Autodesk Inventor part; units mm, degrees
ref_plane "YZ Plane" through (0, 0, 0) normal (1, 0, 0) x (0, 1, 0)
ref_plane "XZ Plane" through (0, 0, 0) normal (0, 1, 0) x (-1, 0, 0)
ref_plane "XY Plane" through (0, 0, 0) normal (0, 0, 1) x (1, 0, 0)
sketch "Skizze1" plane through (0, 0, 0) normal (0, 1, 0) x (-1, 0, 0)
  line L0 (31, 31) -> (-31, 31)
  line L1 (-31, 31) -> (-31, -31)
  line L2 (-31, -31) -> (31, -31)
  line L3 (31, -31) -> (31, 31)
  line L4 (31, 31) -> (-31, -31) construction
  line L5 (-31, 31) -> (31, -31) construction
  point P0 (0, 0)
  dimension "d0" = 62
  dimension "d1" = 62
extrude "Extrusion1" add sketch "Skizze1" along normal blind 2
fillet "Rundung1" radius 6 4 edges at (-31, 1, 31) (31, 1, 31) (31, 1, -31) (-31, 1, -31)
sketch "Skizze2" plane through (0, 2, 0) normal (0, 1, 0) x (1, 0, 0)
  line L0 (-25, -31) -> (25, -31)
  line L1 (0, -31) -> (0, 31) construction
  line L2 (25, 31) -> (-25, 31)
  line L3 (31, -25) -> (31, 25)
  line L4 (31, 0) -> (-31, 0) construction
  line L5 (-31, 25) -> (-31, -25)
  point P0 (0, 0)
  point P1 (21.124, 21.124)
  point P2 (21.124, -21.124)
  point P3 (-21.124, 21.124)
  point P4 (-21.124, -21.124)
  dimension "d37" = 42.248
  dimension "d38" = 42.248
  dimension "d39" = 42.248
hole "Bohrung1" at (21.124, 2, -21.124) at (21.124, 2, 21.124) at (-21.124, 2, -21.124) at (-21.124, 2, 21.124) direction (0, -1, 0) diameter 6 depth 2
hole "Bohrung2" at (0, 2, 0) direction (0, -1, 0) diameter 29 depth 2
sketch "Skizze3" plane through (0, 0, 0) normal (0, -1, 0) x (1, 0, 0)
  point P0 (0, 0)
  point P1 (-14.5, 14.5)
  point P2 (14.5, 14.5)
  point P3 (-14.5, -14.5)
  point P4 (14.5, -14.5)
  dimension "d33" = 29
  dimension "d34" = 14.5
  dimension "d35" = 29
  dimension "d36" = 14.5
hole "Bohrung3" at (-14.5, 0, 14.5) at (14.5, 0, 14.5) at (-14.5, 0, -14.5) at (14.5, 0, -14.5) direction (0, 1, 0) diameter 5 depth 2
properties part number "12"
CAD build for the part. Positions are in the model's coordinates, mm. Round coordinates to 2 decimals unless told otherwise and drop trailing zeros. Write each loop counter-clockwise with the first axis right and the second up, starting at its lowest first coordinate (ties: lowest second). Pieces come first, ordered by that corner, then holes. Notation, with made-up numbers: M 75.25,22 L 131.25,22 A20 cw 131.25,34 Z; hole C 70,8.25 d2. An arc over 180 degrees is marked long. One line per question, with ' | ' between items.
1. Mould opens along X. For faces 1 (the cylindrical face through (29.196, 1.014, 29.289)), 2 (the flat face through (14, 2, 7)), 3 (the cylindrical face through (-21.26, 0.99, -24.12)) say: pulls with the +X half, pulls with the -X half, needs draft (parallel to the pull), parting line crosses it, or undercut.
Working result:
face 1: pulls with the +X half | face 2: needs draft | face 3: undercut
2. Cut at A-A on x = 0. Write the cut outline in (y, z).
Working result:
outline: M 0,-31 L 2,-31 L 2,-14.5 L 0,-14.5 Z; M 0,14.5 L 2,14.5 L 2,31 L 0,31 Z
3. Probe L1, parallel to Z at x = -22, y = 0.9; L2, parallel to X at y = 1.7, z = 19.5; L3, parallel to Z at x = 15, y = 0.1. List the from-to ranges inside material, lowest first. Write a range as from..to.
Working result:
L1: -31..-23.99, -18.25..18.25, 23.99..31 | L2: -31..-23.65, -18.6..18.6, 23.65..31 | L3: -31..-16.95, -12.05..12.05, 16.95..31
4. Cut at C-C on z = 0. Write the cut outline in (x, y), and give its area (3 significant figures).
Working result:
outline: M -31,0 L -14.5,0 L -14.5,2 L -31,2 Z; M 14.5,0 L 31,0 L 31,2 L 14.5,2 Z | area: 66.0 mm2
5. Pin check, flat tip, straight feed: pin 1 Ø6.5 at (x, z) = (14.5, 14.5) entering from -Y. Stop position of the tip, or through.
Working result:
pin 1: y = 0
6. Cut at D-D on z = 13.5. Write the cut outline in (x, y).
Working result:
outline: M -31,0 L -16.79,0 L -16.79,2 L -31,2 Z; M -12.21,0 L -5.29,0 L -5.29,2 L -12.21,2 Z; M 5.29,0 L 12.21,0 L 12.21,2 L 5.29,2 Z; M 16.79,0 L 31,0 L 31,2 L 16.79,2 Z
7. Cut at B-B on x = -16. Write the cut outline in (y, z).
Working result:
outline: M 0,-31 L 2,-31 L 2,-16.5 L 0,-16.5 Z; M 0,-12.5 L 2,-12.5 L 2,12.5 L 0,12.5 Z; M 0,16.5 L 2,16.5 L 2,31 L 0,31 Z
